Model file for the job. Use its own axes, mm. Round coordinates to 2 decimals unless told otherwise and drop trailing zeros. Order: outer loops, then holes, each group sorted by start corner. A loop starts at its lowest first (then second) coordinate and runs counter-clockwise, first axis right, second up. Notation, with made-up numbers: (66.25, 55) -> (104.25, 55) arc R24 cw to (104.25, 68) -> close; hole circle Ø9 at (1, 84). An arc over 180 degrees is marked (long way). Use CSV: the item, a comma, the result in double quotes.
```python
from build123d import *

# Parameters (mm, degrees)
F0_W     = 235
F0_H     = 100
F0_R     = 15
F1_DEPTH = 25
F2_R     = 49.99999


# Not quite as in the source:
# - a fillet or chamfer is up to 0.001 mm smaller than in the source, because OpenCascade refuses the exact size


with BuildPart() as f1:
    # F0 (on Right) → F1 (new body)
    with BuildSketch(Plane.YZ):
        with Locations((67.5, 0)):
            Rectangle(F0_W, F0_H)
        Circle(F0_R, mode=Mode.SUBTRACT)
    extrude(amount=F1_DEPTH)

    # F2 (radius 50 in the source; OpenCascade refuses exactly that, so slightly less here)
    f2_edges = [f1.edges().sort_by_distance(p)[0] for p in [
        (12.5, -50, 50),
        (12.5, -50, -50),
    ]]
    fillet(f2_edges, radius=F2_R)


solid = f1.part
```
Q1. Cut at B-B (z = -12.5). Give the cut face in (x, y).
From the geometry:
outline,"(0, -48.41) -> (25, -48.41) -> (25, -8.29) -> (0, -8.29) -> close; (0, 8.29) -> (25, 8.29) -> (25, 185) -> (0, 185) -> close"
Q2. Cut at C-C (z = -34). Give the cut face in (x, y), plus the area to 3 significant figures.
From the geometry:
outline,"(0, -36.66) -> (25, -36.66) -> (25, 185) -> (0, 185) -> close"
area,"5,540 mm²"
Q3. Pin check, flat tips, straight feed: pin 1 (2 mm diameter, centred on x = 11, y = -5.5, fed in from -Z); pin 2 (6 mm diameter, centred on x = 22, z = 8.5, fed in from -Y). Stop position of each tip, or through.
From the geometry:
pin 1,"stops at z = -49.8"
pin 2,"stops at y = -49.7"
Q4. Cut at D-D (z = -23). Give the cut face in (x, y), plus the area to 3 significant figures.
From the geometry:
outline,"(0, -44.4) -> (25, -44.4) -> (25, 185) -> (0, 185) -> close"
area,"5,730 mm²"
Q5. Probe line 1 along Z through (x, y) = (20.25, 0); line 2 along Y through (x, z) = (1.5, 6.5); line 3 along Y through (x, z) = (10.75, 10). List the from-to ranges inside material, lowest first.
From the geometry:
line 1,"z = -50 to -15, 15 to 50"
line 2,"y = -49.58 to -13.52, 13.52 to 185"
line 3,"y = -48.99 to -11.18, 11.18 to 185"
